The model under review builds one solid part; all positions refer to its coordinate system, in mm. A direction names the side the tool comes from. Coordinates: 2 decimals unless noted, no trailing zeros. Write each loop counter-clockwise with the first axis right and the second up, starting at its lowest first coordinate (ties: lowest second). Pieces come first, ordered by that corner, then holes.
1) Mouldability with a two-part tool opening along X and no side actions: class faces 6 (the flat face through (-40, 5, -17)), 7 (the cylindrical face through (127.493, 2.465, -0.605)), 8 (the flat face through (1, 7, 32.5)) as released by +X, released by -X, zero draft, split by the parting line, or undercut.
2) For line 1 (Z direction, x = -26, y = 8); line 2 (Z direction, x = 9.5, y = 4.25); line 3 (Y direction, x = -75, z = 29), list the stretches that pass through material, from the lowest coordinate up.
3) For P1, Ø4, axis at x = 31.5, y = 2.5, coming from the +Z side; P2, Ø4, axis at y = 4.5, z = -22, coming from the -X side; P3, Ø5, axis at y = 2, z = 7, coming from the -X side, all flat-tipped, find the tip position at first contact; note any pin that passes through.
4) Machinability: for faces 1 (the flat face through (-40, 5, 17)), 2 (the flat face through (-1, 2, -27.5)), 3 (the flat face through (2, 0, 6)), 4 (the flat face through (1, 2, 27.5)), 5 (the cylindrical face through (-127.493, 2.465, 0.605)), which of the approach directions +Z, -Z, +X, -X, +Y, -Y give a long, thin tool a straight path to every point of the face, cutting with its end or side? Answer none if there is none.
5) Add section C-C, the plane x = -115.5. State the section outline as (y, z) points, then the cut area to 3 significant figures.
6) Add section D-D, the plane x = 75. State the section outline as (y, z) points.
7) Add section B-B, the plane z = 0. State the section outline as (x, y) points.
8) Add section A-A, the plane y = 7. State the section outline as (x, z) points.
from build123d import *

# Parameters (mm, degrees)
BOSS_EXTRUDE1_DEPTH = 10
CUT_EXTRUDE1_DEPTH  = 5


with BuildPart() as part:
    # Sketch1 → Boss-Extrude1 (new body)
    with BuildSketch(Plane(origin=(0, 0, 0), x_dir=(1, 0, 0), z_dir=(0, 1, 0))):
        with BuildLine():
            Line((-100, 32.5), (100, 32.5))
            ThreePointArc((100, 32.5), (132.5, 0), (100, -32.5))
            Line((100, -32.5), (-100, -32.5))
            ThreePointArc((-100, -32.5), (-132.5, 0), (-100, 32.5))
        make_face()
        Polygon((0, 21.5), (-40, 21.5), (-40, 12), (0, 12), (50, 12), (50, 21.5), align=None, mode=Mode.SUBTRACT)
        Polygon((-50, 4.75), (0, 4.75), (65, 4.75), (65, -4.75), (0, -4.75), (-50, -4.75), align=None, mode=Mode.SUBTRACT)
        Polygon((0, -12), (-40, -12), (-40, -21.5), (0, -21.5), (50, -21.5), (50, -12), align=None, mode=Mode.SUBTRACT)
    extrude(amount=BOSS_EXTRUDE1_DEPTH)

    # Sketch2 → Cut-Extrude1 (cut)
    with BuildSketch(Plane(origin=(0, 0, 0), x_dir=(1, 0, 0), z_dir=(0, 1, 0))):
        with BuildLine():
            Line((-100, 32.5), (100, 32.5))
            ThreePointArc((100, 32.5), (132.5, 0), (100, -32.5))
            Line((100, -32.5), (-100, -32.5))
            ThreePointArc((-100, -32.5), (-132.5, 0), (-100, 32.5))
        make_face()
        with BuildLine():
            Line((-100, 27.5), (100, 27.5))
            ThreePointArc((100, 27.5), (127.5, 0), (100, -27.5))
            Line((100, -27.5), (-100, -27.5))
            ThreePointArc((-100, -27.5), (-127.5, 0), (-100, 27.5))
        make_face(mode=Mode.SUBTRACT)
    extrude(amount=CUT_EXTRUDE1_DEPTH, mode=Mode.SUBTRACT)


solid = part.part
Geometry results:
1. face 6: undercut
1. face 7: released by +X
1. face 8: zero draft
2. line 1: z = -32.5 to -21.5, -12 to -4.75, 4.75 to 12, 21.5 to 32.5
2. line 2: z = -27.5 to -21.5, -12 to -4.75, 4.75 to 12, 21.5 to 27.5
2. line 3: y = 5 to 10
3. P1: stops at z = 27.5
3. P2: stops at x = -125.57
3. P3: stops at x = -127.13
4. face 1: +Y, -Y
4. face 2: -Z, +X, -X, -Y
4. face 3: +Z, -Z, +X, -X, -Y
4. face 4: +Z, +X, -X, -Y
4. face 5: -X, -Y
5. outline: (0, -22.72) - (5, -22.72) - (5, -28.57) - (10, -28.57) - (10, 28.57) - (5, 28.57) - (5, 22.72) - (0, 22.72) - close
5. area: 513 mm2
6. outline: (0, -27.5) - (5, -27.5) - (5, -32.5) - (10, -32.5) - (10, 32.5) - (5, 32.5) - (5, 27.5) - (0, 27.5) - close
7. outline: (-132.5, 5) - (-127.5, 5) - (-127.5, 0) - (-50, 0) - (-50, 10) - (-132.5, 10) - close; (65, 0) - (127.5, 0) - (127.5, 5) - (132.5, 5) - (132.5, 10) - (65, 10) - close
8. outline: (-100, -32.5) - (100, -32.5) arc R32.5 ccw to (100, 32.5) - (-100, 32.5) arc R32.5 ccw to start; hole (-50, -4.75) - (65, -4.75) - (65, 4.75) - (-50, 4.75) - close; hole (-40, -21.5) - (50, -21.5) - (50, -12) - (-40, -12) - close; hole (-40, 12) - (50, 12) - (50, 21.5) - (-40, 21.5) - close
